Work out the finished part from the listing and answer in its coordinate system (mm). Face numbers are marked on the shaded views. A direction names the side the tool comes from. Coordinates: 2 decimals unless noted, no trailing zeros. Order: outer loops, then holes, each group sorted by start corner. A loop starts at its lowest first (then second) coordinate and runs counter-clockwise, first axis right, second up. Notation, with made-up numbers: M 32,22 L 44,22 A26 ccw 44,61 Z; hole C 26.25,-3 d4. An arc over 180 degrees is marked long. Use a Markdown table: item, result.
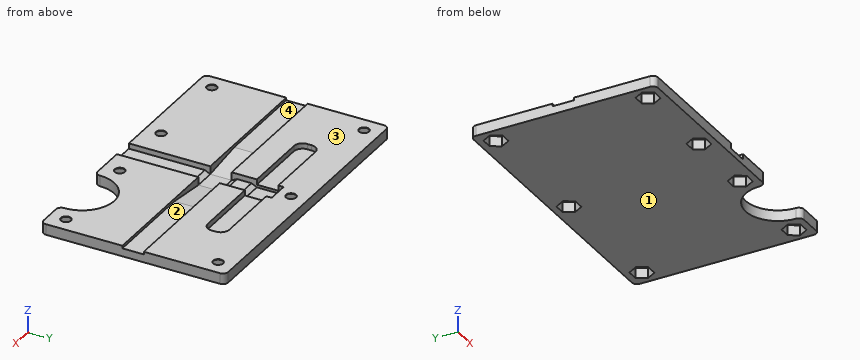
from build123d import *
from OCP.BRepFilletAPI import BRepFilletAPI_MakeChamfer

# Parameters (mm, degrees)
SKETCH1_R           = 1.5
BOSS_EXTRUDE1_DEPTH = 3.175
SKETCH2_W           = 86.995
SKETCH2_H           = 6.35
CUT_EXTRUDE1_DEPTH  = 0.79375
SKETCH3_W           = 6.35
SKETCH3_H           = 30.48
CUT_EXTRUDE2_DEPTH  = 1.5875
SKETCH4_W           = 6.35
SKETCH4_H           = 15.39875
CUT_EXTRUDE3_DEPTH  = 1.5875
SKETCH6_W           = 6.35
SKETCH6_H           = 6.35
CUT_EXTRUDE4_DEPTH  = 0.79375
CHAMFER2_SIZE       = 1.5875
CHAMFER2_SIZE_2     = 0.79375
CUT_EXTRUDE5_DEPTH  = 1.5875
CUT_EXTRUDE6_DEPTH  = 3
SKETCH11_W          = 6.35
SKETCH11_H          = 6.35
CUT_EXTRUDE8_DEPTH  = 0.79375
CHAMFER3_START      = 22.750484618
CHAMFER3_DEPTH      = 6.35
CHAMFER4_SIZE       = 0.79375
CHAMFER4_SIZE_2     = 1.5875


with BuildPart() as part:
    # Sketch1 → Boss-Extrude1 (new body)
    with BuildSketch(Plane.XY.offset(1.6)):
        with BuildLine():
            Line((-17.641226071, 51.730484618), (-17.641226071, 0.120484618))
            ThreePointArc((-17.641226071, 0.120484618), (-17.201886242, -0.940175553), (-16.141226071, -1.379515382))
            Line((-16.141226071, -1.379515382), (39.191273929, -1.379515382))
            ThreePointArc((39.191273929, -1.379515382), (40.313805944, -0.914547397), (40.778773929, 0.207984618))
            ThreePointArc((40.778773929, 0.207984618), (50.303773929, 9.732984618), (59.828773929, 0.207984618))
            ThreePointArc((59.828773929, 0.207984618), (60.293741914, -0.914547397), (61.416273929, -1.379515382))
            Line((61.416273929, -1.379515382), (67.853773929, -1.379515382))
            ThreePointArc((67.853773929, -1.379515382), (68.914434101, -0.940175553), (69.353773929, 0.120484618))
            Line((69.353773929, 0.120484618), (69.353773929, 51.730484618))
            ThreePointArc((69.353773929, 51.730484618), (68.914434101, 52.79114479), (67.853773929, 53.230484618))
            Line((67.853773929, 53.230484618), (-16.141226071, 53.230484618))
            ThreePointArc((-16.141226071, 53.230484618), (-17.201886242, 52.79114479), (-17.641226071, 51.730484618))
        make_face()
        with Locations(Location((-12.878726071, 48.467984618, 0), (0, 0, 180))):
            Circle(SKETCH1_R, mode=Mode.SUBTRACT)
        with Locations(Location((-12.878726071, 3.382984618, 0), (0, 0, 180))):
            Circle(SKETCH1_R, mode=Mode.SUBTRACT)
        with Locations(Location((64.591273929, 3.382984618, 0), (0, 0, 180))):
            Circle(SKETCH1_R, mode=Mode.SUBTRACT)
        with Locations(Location((64.591273929, 48.467984618, 0), (0, 0, 180))):
            Circle(SKETCH1_R, mode=Mode.SUBTRACT)
        with Locations(Location((14.108773929, 3.382984618, 0), (0, 0, 180))):
            Circle(SKETCH1_R, mode=Mode.SUBTRACT)
        with Locations(Location((36.016273929, 3.382984618, 0), (0, 0, 180))):
            Circle(SKETCH1_R, mode=Mode.SUBTRACT)
        with Locations(Location((25.856273929, 48.467984618, 0), (0, 0, 180))):
            Circle(SKETCH1_R, mode=Mode.SUBTRACT)
    extrude(amount=-BOSS_EXTRUDE1_DEPTH)

    # Sketch2 → Cut-Extrude1 (cut)
    with BuildSketch(Plane.XY.offset(1.6)):
        with Locations((25.856273929, 25.925484618)):
            Rectangle(SKETCH2_W, SKETCH2_H)
    extrude(amount=-CUT_EXTRUDE1_DEPTH, mode=Mode.SUBTRACT)

    # Sketch3 → Cut-Extrude2 (cut)
    with BuildSketch(Plane.XY.offset(1.6)):
        with Locations((25.856273929, 13.860484618)):
            Rectangle(SKETCH3_W, SKETCH3_H)
    extrude(amount=-CUT_EXTRUDE2_DEPTH, mode=Mode.SUBTRACT)

    # Sketch4 → Cut-Extrude3 (cut)
    with BuildSketch(Plane.XY.offset(1.6)):
        with Locations((25.856273929, 36.799859618)):
            Rectangle(SKETCH4_W, SKETCH4_H)
    extrude(amount=-CUT_EXTRUDE3_DEPTH, mode=Mode.SUBTRACT)

    # Sketch6 → Cut-Extrude4 (cut)
    with BuildSketch(Plane.XY.offset(0.0125)):
        with Locations((25.856273929, 39.736734618)):
            Rectangle(SKETCH6_W, SKETCH6_H)
    extrude(amount=-CUT_EXTRUDE4_DEPTH, mode=Mode.SUBTRACT)

    # Chamfer2
    chamfer2_edges_1 = [part.edges().sort_by_distance(p)[0] for p in [
        (25.856273929, 36.561734618, 0.0125),
    ]]
    chamfer2_side_1 = [part.faces().sort_by_distance(p)[0] for p in [
        (25.856273929, 36.545859618, 0.0125),
    ]]
    chamfer2_edges_2 = [part.edges().sort_by_distance(p)[0] for p in [
        (25.856273929, 42.911734618, 0.0125),
    ]]
    chamfer2_side_2 = [part.faces().sort_by_distance(p)[0] for p in [
        (25.856273929, 42.927609618, 0.0125),
    ]]
    chamfer2 = BRepFilletAPI_MakeChamfer(part.part.solid().wrapped)
    for e in chamfer2_edges_1:
        chamfer2.Add(CHAMFER2_SIZE - 0.0001, CHAMFER2_SIZE_2 - 0.0001, e.wrapped, chamfer2_side_1[0].wrapped)
    for e in chamfer2_edges_2:
        chamfer2.Add(CHAMFER2_SIZE - 0.0001, CHAMFER2_SIZE_2 - 0.0001, e.wrapped, chamfer2_side_2[0].wrapped)
    add(Compound.cast(chamfer2.Shape()), mode=Mode.REPLACE)  # a hair under: the kernel refuses the full size

    # Sketch7 → Cut-Extrude5 (cut)
    with BuildSketch(Plane.XY.offset(1.6)):
        with BuildLine():
            Line((48.716273929, 42.911734618), (2.996273929, 42.911734618))
            ThreePointArc((2.996273929, 42.911734618), (1.200222705, 42.167785843), (0.456273929, 40.371734618))
            Line((0.456273929, 40.371734618), (0.456273929, 39.101734618))
            ThreePointArc((0.456273929, 39.101734618), (1.200222705, 37.305683394), (2.996273929, 36.561734618))
            Line((2.996273929, 36.561734618), (48.716273929, 36.561734618))
            ThreePointArc((48.716273929, 36.561734618), (50.512325153, 37.305683394), (51.256273929, 39.101734618))
            Line((51.256273929, 39.101734618), (51.256273929, 40.371734618))
            ThreePointArc((51.256273929, 40.371734618), (50.512325153, 42.167785843), (48.716273929, 42.911734618))
        make_face()
    extrude(amount=-CUT_EXTRUDE5_DEPTH, mode=Mode.SUBTRACT)

    # Sketch9 → Cut-Extrude6 (cut)
    with BuildSketch(Plane(origin=(0, 0, -1.575), x_dir=(-1, 0, 0), z_dir=(0, 0, -1))):
        Polygon((-22.623145199, 48.453426307), (-24.227101696, 51.260677077), (-27.460230427, 51.275235389), (-29.08940266, 48.48254293), (-27.485446162, 45.67529216), (-24.252317432, 45.660733848), align=None)
        Polygon((-10.875621178, 3.375460135), (-12.48568116, 6.179214794), (-15.718833912, 6.186739277), (-17.341926681, 3.390509102), (-15.731866699, 0.586754443), (-12.498713947, 0.57922996), align=None)
        Polygon((16.111859882, 3.369602212), (14.50688248, 6.17626943), (11.273748669, 6.189651836), (9.645592259, 3.396367025), (11.250569661, 0.589699807), (14.483703473, 0.576317401), align=None)
        Polygon((16.1118088, 48.445414775), (14.514813493, 51.256631473), (11.281730764, 51.279201317), (9.645643341, 48.490554462), (11.242638648, 45.679337764), (14.475721377, 45.65676792), align=None)
        Polygon((-61.358112429, 48.468201712), (-62.974881187, 51.268093159), (-66.208042688, 51.267876066), (-67.824435429, 48.467767525), (-66.207666671, 45.667876078), (-62.974505171, 45.668093171), align=None)
        Polygon((-61.358112422, 3.382984618), (-62.974693176, 6.182984618), (-66.207854683, 6.182984618), (-67.824435437, 3.382984618), (-66.207854683, 0.582984618), (-62.974693176, 0.582984618), align=None)
        Polygon((-32.784301689, 3.295298985), (-34.324349823, 6.138111866), (-37.556322063, 6.2257975), (-39.24824617, 3.470670252), (-37.708198036, 0.627857371), (-34.476225796, 0.540171737), align=None)
    extrude(amount=-CUT_EXTRUDE6_DEPTH, mode=Mode.SUBTRACT)

    # Sketch11 → Cut-Extrude8 (cut)
    with BuildSketch(Plane.XY.offset(0.0125)):
        with Locations((25.856273929, 25.925484618)):
            Rectangle(SKETCH11_W, SKETCH11_H)
    extrude(amount=-CUT_EXTRUDE8_DEPTH, mode=Mode.SUBTRACT)

    # Chamfer3: read off the stored shape, not the designer's step
    # Chamfer3 outline → Chamfer3 (cut)
    with BuildSketch(Plane(origin=(0, 0, 0), x_dir=(1, 0, 0), z_dir=(0, 1, 0)).offset(CHAMFER3_START)):
        Polygon((22.681273929, 0.78125), (9.981273929, -0.80625), (22.681273929, -0.80625), align=None)
        Polygon((41.731273929, -0.80625), (29.031273929, 0.78125), (29.031273929, -0.80625), align=None)
    extrude(amount=CHAMFER3_DEPTH, mode=Mode.SUBTRACT)

    # Chamfer4
    chamfer4_edges_1 = [part.edges().sort_by_distance(p)[0] for p in [
        (25.856273929, 22.750484618, 0.0125),
    ]]
    chamfer4_side_1 = [part.faces().sort_by_distance(p)[0] for p in [
        (25.856273929, 22.750484618, -0.003375),
    ]]
    chamfer4_edges_2 = [part.edges().sort_by_distance(p)[0] for p in [
        (25.856273929, 29.100484618, 0.0125),
    ]]
    chamfer4_side_2 = [part.faces().sort_by_distance(p)[0] for p in [
        (25.856273929, 29.100484618, -0.003375),
    ]]
    chamfer4 = BRepFilletAPI_MakeChamfer(part.part.solid().wrapped)
    for e in chamfer4_edges_1:
        chamfer4.Add(CHAMFER4_SIZE - 0.0001, CHAMFER4_SIZE_2 - 0.0001, e.wrapped, chamfer4_side_1[0].wrapped)
    for e in chamfer4_edges_2:
        chamfer4.Add(CHAMFER4_SIZE - 0.0001, CHAMFER4_SIZE_2 - 0.0001, e.wrapped, chamfer4_side_2[0].wrapped)
    add(Compound.cast(chamfer4.Shape()), mode=Mode.REPLACE)  # a hair under: the kernel refuses the full size


solid = part.part
1. Section A-A on y = 26.5 is taken. Determine the outline of the cut face in (x, z) (3 decimals).
Answers below:
| item | result |
|---|---|
| outline | M -17.641,-1.575 L 69.354,-1.575 L 69.354,0.806 L 41.731,0.806 L 29.031,-0.781 L 22.681,-0.781 L 9.981,0.806 L -17.641,0.806 Z |
2. Section C-C on y = 18 is taken. Determine the outline of the cut face in (x, z) (1 decimal), then the cut area to 3 significant figures.
Answers below:
| item | result |
|---|---|
| outline | M -17.6,-1.6 L 69.4,-1.6 L 69.4,1.6 L 29,1.6 L 29,0 L 22.7,0 L 22.7,1.6 L -17.6,1.6 Z |
| area | 266 mm² |
3. For the marked faces 3 and 4, determine the directions among +Z, -Z, +X, -X, +Y, -Y from which every point of the face is accessible in a straight line to the end or side of a thin tool.
Answers below:
| item | result |
|---|---|
| face 3 | +Z, +X, -X, +Y, -Y |
| face 4 | +Z, +X, -X |
4. Find the intervals of material crossed by probe 1 along Y at (x, z) = (15, -0.6); probe 2 along Y at (x, z) = (61.5, 1.35); probe 3 along Y at (x, z) = (24.5, 1.05), in increasing order.
Answers below:
| item | result |
|---|---|
| probe 1 | -1.38 to 0.59, 6.19 to 53.23 |
| probe 2 | -1.38 to 3.14, 3.63 to 22.75, 29.1 to 48.22, 48.71 to 53.23 |
| probe 3 | 44.5 to 45.66, 51.26 to 53.23 |
5. For a pull along Y with two mould halves and no side action, classify the marked faces 1 and 2 as +Y half, -Y half, draft (parallel to the pull), parting line (faces both ways), or undercut.
Answers below:
| item | result |
|---|---|
| face 1 | draft |
| face 2 | undercut |
6. Section B-B on x = 4 is taken. Determine the outline of the cut face in (y, z) (1 decimal), then the cut area to 3 significant figures.
Answers below:
| item | result |
|---|---|
| outline | M -1.4,-1.6 L 53.2,-1.6 L 53.2,1.6 L 42.9,1.6 L 42.9,0 L 36.6,0 L 36.6,1.6 L 29.1,1.6 L 29.1,0.8 L 22.8,0.8 L 22.8,1.6 L -1.4,1.6 Z |
| area | 158 mm² |
7. Flat-ended cylindrical pins translate along their axes: P1, Ø3, axis at x = 41.5, y = 41, coming from the +Z side; P2, Ø1.7, axis at x = 14, y = 4.5, coming from the -Z side (3 decimals); P3, Ø3, axis at x = 55.5, y = 24.5, coming from the +Z side. Find the tip coordinate at first contact, or state that the pin passes through.
Answers below:
| item | result |
|---|---|
| P1 | z = 0.01 |
| P2 | z = 1.425 |
| P3 | z = 0.81 |
8. Section D-D on y = 42 is taken. Determine the outline of the cut face in (x, z) (1 decimal), then the cut area to 3 significant figures.
Answers below:
| item | result |
|---|---|
| outline | M -17.6,-1.6 L 69.4,-1.6 L 69.4,1.6 L 50.7,1.6 L 50.7,0 L 29,0 L 29,-0.8 L 22.7,-0.8 L 22.7,0 L 1,0 L 1,1.6 L -17.6,1.6 Z |
| area | 192 mm² |
